The listing builds one solid part. Answer for the finished solid, in the listing's coordinates (mm). A direction names the side the tool comes from. Coordinates: 2 decimals unless noted, no trailing zeros. Order: outer loops, then holes, each group sorted by start corner. A loop starts at its lowest first (then second) coordinate and runs counter-clockwise, first axis right, second up. Notation, with made-up numbers: (81.5, 13.5) - (106.5, 13.5) arc R33 cw to (106.5, 50.5) - close; hole circle Ø8 at (39, 83). An arc over 180 degrees is marked (long way). Use a Markdown table: item, result. Add a question column.
Item 1: The part is cut by section A-A, the plane z = 4.65. State how many separate pieces and enclosed holes the cut face has, then the cut area to 3 significant figures.
Item 2: For faces 4 (the flat face through (-5, 7.485, 3)), 5 (the flat face through (8, 3.81, 3)), 6 (the flat face through (0, -4, 0)), determine the directions among +Z, -Z, +X, -X, +Y, -Y from which every point of the face is accessible in a straight line to the end or side of a thin tool.
Item 3: The part is cut by section C-C, the plane y = 2.5. Give the vertices of the cut face in (x, z), then the cut area to 3 significant figures.
Item 4: Find the intervals of material crossed by line 1 along Y through (x, z) = (0, 1.9) (3 decimals); line 2 along Y through (x, z) = (-6, 2.8) (3 decimals); line 3 along X through (y, z) = (1, 2.95), in increasing order.
Item 5: The part is cut by section D-D, the plane x = 6.5. Give the vertices of the cut face in (y, z).
Item 6: Flat-ended cylindrical pins translate along their axes: P1, Ø3, axis at x = 8.5, z = 3.5, coming from the +Y side; P2, Ø3, axis at x = -5.5, z = 3, coming from the -Y side; P3, Ø3, axis at y = 5.5, z = 3.5, coming from the +X side; P4, Ø1, axis at x = 12.5, y = 11.5, coming from the -Z side. Find the tip coordinate at first contact, or state that the pin passes through.
Item 7: The mould has two halves that part along X. Classify faces 1 (the flat face through (0, -4, 5.8)), 2 (the cylindrical face through (7.25, 0.05, 2.86)), 3 (the cylindrical face through (-15.64, 5.79, 2.86)): released by +X, released by -X, zero draft, split by the parting line, or undercut.
Item 8: The part is cut by section B-B, the plane x = 0. Give the vertices of the cut face in (y, z) (3 decimals), then the cut area to 3 significant figures.
from build123d import *

# Parameters (mm, degrees)
SKETCH1_R                 = 17.229166667
SKETCH1_R_2               = 3
BOSS_EXTRUDE1_DEPTH       = 5.8
SKETCH2_R                 = 0.79375
CUT_EXTRUDE1_DEPTH        = 26.046524071
CUT_EXTRUDE2_DEPTH        = 26.046524071
FILLET1_R                 = 3.175
FILLET2_R                 = 0.508
M3X0_5_TAPPED_HOLE1_D     = 2.5
M3X0_5_TAPPED_HOLE1_DEPTH = 8.636
M3X0_5_TAPPED_HOLE1_TIP   = 0.751075774


with BuildPart() as part:
    # Sketch1 → Boss-Extrude1 (new body)
    with BuildSketch(Plane.XY):
        Circle(SKETCH1_R)
        Circle(SKETCH1_R_2, mode=Mode.SUBTRACT)
    extrude(amount=BOSS_EXTRUDE1_DEPTH)

    # Sketch2 → Cut-Extrude1 (cut, through all)
    with BuildSketch(Plane.XY.offset(5.8)):
        with Locations((0, 12)):
            Circle(SKETCH2_R)
        with Locations((12, 0)):
            Circle(SKETCH2_R)
        with Locations((0, -12)):
            Circle(SKETCH2_R)
        with Locations((-12, 0)):
            Circle(SKETCH2_R)
    extrude(amount=-CUT_EXTRUDE1_DEPTH, mode=Mode.SUBTRACT)

    # Sketch3 → Cut-Extrude2 (cut, through all)
    with BuildSketch(Plane.XY.offset(5.8)):
        with BuildLine():
            Line((-15.518342664, 7.485), (4.357889894, 7.485))
            Line((4.357889894, 7.485), (4.357889894, 10.16))
            Line((4.357889894, 10.16), (10.707889894, 10.16))
            Line((10.707889894, 10.16), (10.707889894, 3.81))
            Line((10.707889894, 3.81), (4.357889894, 3.81))
            Line((4.357889894, 3.81), (4.357889894, 6.485))
            Line((4.357889894, 6.485), (-15.962110106, 6.485))
            ThreePointArc((-15.962110106, 6.485), (-15.748165818, 6.988523262), (-15.518342664, 7.485))
        make_face()
    extrude(amount=-CUT_EXTRUDE2_DEPTH, mode=Mode.SUBTRACT)

    # Fillet1
    fillet1_edges = [part.edges().sort_by_distance(p)[0] for p in [
        (-15.962110106, 6.485, 2.9),
    ]]
    fillet(fillet1_edges, radius=FILLET1_R)

    # Fillet2
    fillet2_edges = [part.edges().sort_by_distance(p)[0] for p in [
        (-15.518342664, 7.485, 2.9),
    ]]
    fillet(fillet2_edges, radius=FILLET2_R)

    # M3x0.5 Tapped Hole1
    with Locations(Plane.XY.offset(5.8)):
        with Locations((-6, 0), (6, 0)):
            Hole(M3X0_5_TAPPED_HOLE1_D / 2, depth=M3X0_5_TAPPED_HOLE1_DEPTH)
            with Locations((0, 0, -(M3X0_5_TAPPED_HOLE1_DEPTH + M3X0_5_TAPPED_HOLE1_TIP / 2))):  # 118° drill point
                Cone(0, M3X0_5_TAPPED_HOLE1_D / 2, M3X0_5_TAPPED_HOLE1_TIP, mode=Mode.SUBTRACT)


solid = part.part
Solution:
| question | item | result |
|---|---|---|
| 1 | separate pieces | 1 |
| 1 | enclosed holes | 7 |
| 1 | area | 825 mm2 |
| 2 | face 4 | +Z, -Z, -X |
| 2 | face 5 | +Z, -Z |
| 2 | face 6 | -Z, +X, -X, +Y, -Y |
| 3 | outline | (-17.05, 0) - (-1.66, 0) - (-1.66, 5.8) - (-17.05, 5.8) - close; (1.66, 0) - (17.05, 0) - (17.05, 5.8) - (1.66, 5.8) - close |
| 3 | area | 179 mm2 |
| 4 | line 1 | y = -17.229 to -12.794, -11.206 to -3, 3 to 6.485, 7.485 to 11.206, 12.794 to 17.229 |
| 4 | line 2 | y = -16.151 to -1.25, 1.25 to 6.485, 7.485 to 16.151 |
| 4 | line 3 | x = -17.2 to -6.75, -5.25 to -2.83, 2.83 to 5.25, 6.75 to 17.2 |
| 5 | outline | (-15.96, 0) - (-1.15, 0) - (-1.15, 5.8) - (-15.96, 5.8) - close; (1.15, 0) - (3.81, 0) - (3.81, 5.8) - (1.15, 5.8) - close; (10.16, 0) - (15.96, 0) - (15.96, 5.8) - (10.16, 5.8) - close |
| 6 | P1 | stops at y = 15.74 |
| 6 | P2 | stops at y = -16.76 |
| 6 | P3 | stops at x = 16.76 |
| 6 | P4 | stops at z = 0 |
| 7 | face 1 | zero draft |
| 7 | face 2 | undercut |
| 7 | face 3 | released by -X |
| 8 | outline | (-17.229, 0) - (-12.794, 0) - (-12.794, 5.8) - (-17.229, 5.8) - close; (-11.206, 0) - (-3, 0) - (-3, 5.8) - (-11.206, 5.8) - close; (3, 0) - (6.485, 0) - (6.485, 5.8) - (3, 5.8) - close; (7.485, 0) - (11.206, 0) - (11.206, 5.8) - (7.485, 5.8) - close; (12.794, 0) - (17.229, 0) - (17.229, 5.8) - (12.794, 5.8) - close |
| 8 | area | 141 mm2 |
